Work out the finished part from the listing and answer in its coordinate system (mm). Face numbers are marked on the shaded views. A direction names the side the tool comes from. Coordinates: 2 decimals unless noted, no trailing zeros. Loops run counter-clockwise (first coordinate to the right, second up) from the corner with the lowest first, then second, coordinate; pieces in that order, holes last. Notation, with made-up numbers: (78, 67.25) -> (136, 67.25) arc R34 cw to (136, 101.25) -> close; hole circle Ø11 at (82, 29.25). An arc over 180 degrees is marked (long way). Answer as CSV lines item,"result".
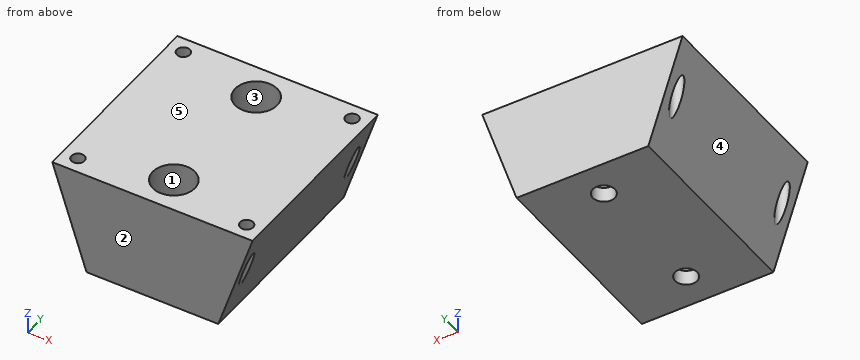
Autodesk Inventor part; units mm, degrees
ref_plane "YZ Plane" through (0, 0, 0) normal (1, 0, 0) x (0, 1, 0)
ref_plane "XZ Plane" through (0, 0, 0) normal (0, 1, 0) x (-1, 0, 0)
ref_plane "XY Plane" through (0, 0, 0) normal (0, 0, 1) x (1, 0, 0)
sketch "Sketch1" plane through (0, 0, 0) normal (0, 0, 1) x (1, 0, 0)
  line L0 (12.5, -19) -> (-12.5, -19)
  line L1 (-12.5, -19) -> (-12.5, 19)
  line L2 (-12.5, 19) -> (12.5, 19)
  line L3 (12.5, 19) -> (12.5, -19)
  line L4 (12.5, -19) -> (-12.5, 19) construction
  line L5 (-12.5, -19) -> (12.5, 19) construction
  circle A0 centre (0, 12.5) radius 2.1
  circle A1 centre (0, -12.5) radius 2.1
  point P0 (0, 0)
  dimension "d0" = 25
  dimension "d1" = 38
  dimension "d2" = 4.2
  dimension "d3" = 4.2
  dimension "d4" = 12.5
  dimension "d5" = 12.5
extrude "Extrusion1" add sketch "Sketch1" along normal blind 20
sketch "Sketch2" plane through (-12.5, 19, 0) normal (0, 1, 0) x (1, 0, 0)
  line L0 (0, 0) -> (0, -20)
  line L1 (0, -20) -> (-6.5, -20)
  line L2 (-6.5, -20) -> (0, 0)
  line L3 (0, -20) -> (25, -20)
  line L4 (0, 0) -> (0, -20)
  line L5 (25, -20) -> (31.5, -20)
  line L6 (25, 0) -> (25, -20)
  line L7 (31.5, -20) -> (25, 0)
  line L8 (25, 0) -> (25, -20)
  point P0 (12.5, 0)
  dimension "d8" = 6.5
  dimension "d9" = 6.5
extrude "Extrusion2" add sketch "Sketch2" against normal up to surface (38 mm away)
sketch "Sketch3" plane through (0, 0, 20) normal (0, 0, 1) x (1, 0, 0)
  line L0 (-5.4088, 0) -> (7.7062, 0)
  line L1 (0, 5.8117) -> (0, -6.6687)
  point P0 (0, 0)
  point P1 (-16, 16)
  point P2 (16, 16)
  point P3 (-16, -16)
  point P4 (16, -16)
  dimension "d12" = 16
  dimension "d13" = 16
  dimension "d16" = 32
  dimension "d19" = 32
hole "Hole1" at (-16, 16, 20) at (16, 16, 20) at (-16, -16, 20) at (16, -16, 20) direction (0, 0, -1) diameter 2.5 end through all
hole "Hole2" at (0, -12.5, 20) direction (0, 0, -1) diameter 8 depth 16 tip angle 118
hole "Hole3" at (0, 12.5, 20) direction (0, 0, -1) diameter 8 depth 16 tip angle 118
properties part number "RDtoRC2-height20mm"
(1) Consider line 1 along Y through (x, z) = (0, 2.15); line 2 along Y through (x, z) = (16, 15.25); line 3 along X through (y, z) = (-16, 15.75). Determine where each line is inside the solid, lowest interval first.
Computed values:
line 1,"-19 to -14.6, -10.4 to 10.4, 14.6 to 19"
line 2,"-19 to -17.25, -14.75 to 14.75, 17.25 to 19"
line 3,"-17.62 to -17.25, -14.75 to -1.94, 1.94 to 14.75, 17.25 to 17.62"
(2) A cutting plane is placed at C-C, the plane y = -12.5. Write down the section's boundary in (x, z).
Computed values:
outline,"(-19, 20) -> (-12.5, 0) -> (-2.1, 0) -> (-2.1, 2.86) -> (-4, 4) -> (-4, 20) -> close; (2.1, 0) -> (12.5, 0) -> (19, 20) -> (4, 20) -> (4, 4) -> (2.1, 2.86) -> close"
(3) Which of the six approach directions +Z, -Z, +X, -X, +Y, -Y give full straight-line access (tool end or side, diameter ignored) to the marked faces 1 and 2?
Computed values:
face 1,"+Z"
face 2,"+Z, -Z, +X, -X, -Y"
(4) A cutting plane is placed at D-D, the plane y = -7.5. Write down the section's boundary in (x, z), and give its area (3 significant figures).
Computed values:
outline,"(-19, 20) -> (-12.5, 0) -> (12.5, 0) -> (19, 20) -> close"
area,"630 mm2"
(5) For a pull along X with two mould halves and no side action, classify the marked faces 3, 4 and 5 as pulls with the +X half, pulls with the -X half, needs draft (parallel to the pull), parting line crosses it, or undercut.
Computed values:
face 3,"undercut"
face 4,"pulls with the -X half"
face 5,"needs draft"
(6) A cutting plane is placed at B-B, the plane z = 18. Write down the section's boundary in (x, y), and give its area (3 significant figures).
Computed values:
outline,"(-18.35, -19) -> (18.35, -19) -> (18.35, 19) -> (-18.35, 19) -> close; hole circle Ø2.5 at (-16, -16); hole circle Ø2.5 at (-16, 16); hole circle Ø8 at (0, -12.5); hole circle Ø8 at (0, 12.5); hole circle Ø2.5 at (16, -16); hole circle Ø2.5 at (16, 16)"
area,"1,270 mm2"
(7) Flat-ended cylindrical pins translate along their axes: pin 1 Ø3 at (x, y) = (16, -16) entering from +Z; pin 2 Ø12 at (y, z) = (12, 12.5) entering from +X; pin 3 Ø5 at (y, z) = (9.5, 4.5) entering from +X (3 decimals). Find the tip coordinate at first contact, or state that the pin passes through.
Computed values:
pin 1,"z = 20"
pin 2,"x = 18.51"
pin 3,"x = 14.775"
(8) A cutting plane is placed at A-A, the plane x = 0. Write down the section's boundary in (y, z).
Computed values:
outline,"(-19, 0) -> (-14.6, 0) -> (-14.6, 2.86) -> (-16.5, 4) -> (-16.5, 20) -> (-19, 20) -> close; (-10.4, 0) -> (10.4, 0) -> (10.4, 2.86) -> (8.5, 4) -> (8.5, 20) -> (-8.5, 20) -> (-8.5, 4) -> (-10.4, 2.86) -> close; (14.6, 0) -> (19, 0) -> (19, 20) -> (16.5, 20) -> (16.5, 4) -> (14.6, 2.86) -> close"
